from build123d import *

# Parameters (mm, degrees)
F0_W     = 254
F0_H     = 203.2
F1_DEPTH = 12.7
F4_DEPTH = 254.001
F2_W     = 50.8
F2_H     = 12.7
F5_DEPTH = 12.701


with BuildPart() as f1:
    # F0 (on Top) → F1 (new body)
    with BuildSketch(Plane.XY):
        Rectangle(F0_W, F0_H)
    extrude(amount=F1_DEPTH)

    # F3 (on face) → F4 (cut, through all)
    with BuildSketch(Plane(origin=(-127, 0, 0), x_dir=(0, -1, 0), z_dir=(-1, 0, 0))):
        with BuildLine():
            ThreePointArc((-92.075, 6.35), (-95.25, 9.525), (-98.425, 6.35))
            Line((-98.425, 6.35), (-92.075, 6.35))
        make_face()
        with BuildLine():
            Line((-92.075, 6.35), (-98.425, 6.35))
            ThreePointArc((-98.425, 6.35), (-95.25, 3.175), (-92.075, 6.35))
        make_face()
    extrude(amount=-F4_DEPTH, mode=Mode.SUBTRACT)

    # F2 (on face) → F5 (cut, through all)
    with BuildSketch(Plane.XY.offset(12.7)):
        with Locations((-101.6, 95.25)):
            Rectangle(F2_W, F2_H)
        with Locations((101.6, 95.25)):
            Rectangle(F2_W, F2_H)
    extrude(amount=-F5_DEPTH, mode=Mode.SUBTRACT)


solid = f1.part
For this review, take the finished solid that the model builds, in its own axes (mm). A direction names the side the tool comes from. Round coordinates to 2 decimals unless told otherwise and drop trailing zeros. Loops run counter-clockwise (first coordinate to the right, second up) from the corner with the lowest first, then second, coordinate; pieces in that order, holes last. Notation, with made-up numbers: (4, -8.5) - (58, -8.5) arc R16 ccw to (58, 6.5) - close; hole circle Ø4 at (-5, -11). An arc over 180 degrees is marked (long way). Use one line per item in the form item = value.
Item 1: Clearance check with flat-ended pins moving along their axes: P1, Ø4, axis at y = 95.5, z = 7, coming from the -X side; P2, Ø4, axis at x = -113, z = 3.5, coming from the +Y side. State where each tip first meets the part, or that it passes through.
Answers:
P1 = through
P2 = 88.9
Item 2: Tool access review of faces 4 (the flat face through (76.2, 92, 8)), 5 (the flat face through (-2, 1, 0)), 6 (the flat face through (-76.2, 92, 8)): name each direction out of +Z, -Z, +X, -X, +Y, -Y from which nothing blocks a thin tool from reaching the whole face with its end or side.
Answers:
face_4 = +Z, -Z, +X, +Y
face_5 = -Z, +X, -X, +Y, -Y
face_6 = +Z, -Z, -X, +Y
Item 3: Consider section A-A on y = 95.25. Write out the cut boundary in (x, z) (3 decimals), then the cut area to 3 significant figures.
Answers:
outline = (-76.2, 0) - (76.2, 0) - (76.2, 3.175) - (-76.2, 3.175) - close; (-76.2, 9.525) - (76.2, 9.525) - (76.2, 12.7) - (-76.2, 12.7) - close
area = 968 mm^2
Item 4: For line 1 (Y direction, x = 7, z = 6.5); line 2 (Z direction, x = 42, y = 95); line 3 (Y direction, x = 108.5, z = 3.5), list the stretches that pass through material, from the lowest coordinate up.
Answers:
line_1 = -101.6 to 92.08, 98.42 to 101.6
line_2 = 0 to 3.18, 9.52 to 12.7
line_3 = -101.6 to 88.9
Item 5: Consider section B-B on z = 6.35. Write out the cut boundary in (x, y) (3 decimals), then the cut area to 3 significant figures.
Answers:
outline = (-127, -101.6) - (127, -101.6) - (127, 88.9) - (76.2, 88.9) - (76.2, 92.075) - (-76.2, 92.075) - (-76.2, 88.9) - (-127, 88.9) - close; (-76.2, 98.425) - (76.2, 98.425) - (76.2, 101.6) - (-76.2, 101.6) - close
area = 49,400 mm^2
Item 6: Mouldability with a two-part tool opening along Z and no side actions: class faces 1 (the cylindrical face through (-1.07, 98.28, 5.4)), 2 (the flat face through (-2, 1, 12.7)), 3 (the flat face through (127, -8, 6)) as +Z half, -Z half, draft (parallel to the pull), parting line (faces both ways), or undercut.
Answers:
face_1 = undercut
face_2 = +Z half
face_3 = draft
Item 7: Consider section C-C on x = -93. Write out the cut boundary in (y, z).
Answers:
outline = (-101.6, 0) - (88.9, 0) - (88.9, 12.7) - (-101.6, 12.7) - close
